Geometry check sheet. Reference: the model listing, model coordinates, mm. Give positions to 0.01 mm unless a question says otherwise; leave off trailing zeros. Write each loop counter-clockwise with the first axis right and the second up, starting at its lowest first coordinate (ties: lowest second). Pieces come first, ordered by that corner, then holes. Notation, with made-up numbers: (51, 58.5) - (103, 58.5) arc R20 ccw to (103, 89.5) - close; hole circle Ø8 at (85.25, 15). An arc over 180 degrees is marked (long way). Use a Markdown table: item, result.
```python
from build123d import *

# Parameters (mm, degrees)
SKETCH1_W               = 76.2
SKETCH1_H               = 76.2
BOSS_EXTRUDE1_DEPTH     = 1.57
CUT_EXTRUDE1_DEPTH      = 16
CUT_EXTRUDE1_DEPTH_BACK = 10.57
SKETCH1_4_R             = 2.159
CUT_EXTRUDE2_DEPTH      = 24
CUT_EXTRUDE2_DEPTH_BACK = 19.57
SKETCH1_5_R             = 2.159
FILLET1_R               = 8


with BuildPart() as part:
    # Sketch1 → Boss-Extrude1 (new body)
    with BuildSketch(Plane.XY):
        Rectangle(SKETCH1_W, SKETCH1_H)
    extrude(amount=BOSS_EXTRUDE1_DEPTH)

    # Sketch1_4 → Cut-Extrude1 (cut, two sides: drawn at the far end of the back side and taken through both)
    with BuildSketch(Plane.XY.offset(-CUT_EXTRUDE1_DEPTH_BACK)):
        with Locations((29.591, 29.591)):
            Circle(SKETCH1_4_R)
    extrude(amount=CUT_EXTRUDE1_DEPTH + CUT_EXTRUDE1_DEPTH_BACK, mode=Mode.SUBTRACT)

    # Sketch1_5 → Cut-Extrude2 (cut, two sides: drawn at the far end of the back side and taken through both)
    with BuildSketch(Plane.XY.offset(-CUT_EXTRUDE2_DEPTH_BACK)):
        with Locations((-29.591, 29.591)):
            Circle(SKETCH1_5_R)
        with Locations((-29.591, -29.591)):
            Circle(SKETCH1_5_R)
        with Locations((29.591, -29.591)):
            Circle(SKETCH1_5_R)
    extrude(amount=CUT_EXTRUDE2_DEPTH + CUT_EXTRUDE2_DEPTH_BACK, mode=Mode.SUBTRACT)

    # Fillet1
    fillet1_edges = [part.edges().sort_by_distance(p)[0] for p in [
        (-38.1, 38.1, 0.785),
        (38.1, 38.1, 0.785),
        (38.1, -38.1, 0.785),
        (-38.1, -38.1, 0.785),
    ]]
    fillet(fillet1_edges, radius=FILLET1_R)


solid = part.part
```
1) Section check A-A on z = 0.8. Record the boundary of the cut face in (x, y), then the cut area to 3 significant figures.
Working result:
| item | result |
|---|---|
| outline | (-38.1, -30.1) arc R8 ccw to (-30.1, -38.1) - (30.1, -38.1) arc R8 ccw to (38.1, -30.1) - (38.1, 30.1) arc R8 ccw to (30.1, 38.1) - (-30.1, 38.1) arc R8 ccw to (-38.1, 30.1) - close; hole circle Ø4.32 at (-29.59, -29.59); hole circle Ø4.32 at (-29.59, 29.59); hole circle Ø4.32 at (29.59, -29.59); hole circle Ø4.32 at (29.59, 29.59) |
| area | 5,690 mm² |
2) Material ranges on L1, parallel to X at y = -29.5, z = 0.4; L2, parallel to X at y = -31, z = 0.95; L3, parallel to Y at x = 30.5, z = 0.35, recorded low to high. Write a range as from..to.
Working result:
| item | result |
|---|---|
| L1 | x = -38.1..-31.75, -27.43..27.43, 31.75..38.1 |
| L2 | x = -38.05..-31.23, -27.96..27.96, 31.23..38.05 |
| L3 | y = -38.09..-31.55, -27.63..27.63, 31.55..38.09 |
3) Mould release check, pull along Y, two halves, no side actions. Record for faces 1 (the cylindrical face through (-35.819, 35.694, 0.796)), 2 (the cylindrical face through (-28.59, 27.68, 0.77)), 3 (the cylindrical face through (-35.819, -35.694, 0.796)): pulls with the +Y half, pulls with the -Y half, needs draft (parallel to the pull), parting line crosses it, or undercut.
Working result:
| item | result |
|---|---|
| face 1 | pulls with the +Y half |
| face 2 | undercut |
| face 3 | pulls with the -Y half |
4) Depth check by flat-ended pin: P1, Ø4, axis at x = -29.591, y = -29.591, coming from the +Z side. Enter the tip coordinate at first touch or a pass-through.
Working result:
| item | result |
|---|---|
| P1 | passes through |
